Geometry check sheet. Reference: the model listing, model coordinates, mm. Give positions to 0.01 mm unless a question says otherwise; leave off trailing zeros. Order: outer loops, then holes, each group sorted by start corner. A loop starts at its lowest first (then second) coordinate and runs counter-clockwise, first axis right, second up. Notation, with made-up numbers: M 81.25,-25.75 L 94.25,-25.75 A28 cw 94.25,-2.75 Z; hole C 39,35 d10. An arc over 180 degrees is marked long. Answer as CSV lines item,"result". Start each with the question number.
```python
from build123d import *

# Parameters (mm, degrees)
F0_W     = 50
F0_H     = 70
F0_R     = 3
F1_DEPTH = 8
F2_SIZE  = 2
F3_SIZE  = 5


with BuildPart() as f1:
    # F0 (on Front) → F1 (new body)
    with BuildSketch(Plane.XZ):
        with Locations((-5.015146, 9.995409)):
            Rectangle(F0_W, F0_H)
        with Locations((-10.015146, 4.995409)):
            Circle(F0_R, mode=Mode.SUBTRACT)
        with Locations((11.984854, -17.004591)):
            Circle(F0_R, mode=Mode.SUBTRACT)
        with Locations((8.984854, 4.995409)):
            Circle(F0_R, mode=Mode.SUBTRACT)
        with Locations((11.984854, 36.995409)):
            Circle(F0_R, mode=Mode.SUBTRACT)
    extrude(amount=F1_DEPTH)

    # F2
    f2_edges = [f1.edges().sort_by_distance(p)[0] for p in [
        (-13.015146, -8, 4.995409),
        (5.984854, -8, 4.995409),
    ]]
    chamfer(f2_edges, length=F2_SIZE)

    # F3
    f3_edges = [f1.edges().sort_by_distance(p)[0] for p in [
        (19.984854, -4, 44.995409),
        (19.984854, -4, -25.004591),
        (-30.015146, -4, 44.995409),
        (-30.015146, -4, -25.004591),
    ]]
    chamfer(f3_edges, length=F3_SIZE)


solid = f1.part
```
Item 1: Section check B-B on y = -4.75. Record the boundary of the cut face in (x, z), then the cut area to 3 significant figures.
Item 2: Draft check along X on faces 1 (the face through (-13.14, -6.13, 5.13)), 2 (the face through (-30.015, -4, 10)), 3 (the face through (19.985, -4, 10)). Enter one of: pulls with the +X half, pulls with the -X half, needs draft (parallel to the pull), parting line crosses it, or undercut.
Item 3: Section check A-A on z = -18.5. Record the boundary of the cut face in (x, y), then the cut area to 3 significant figures.
Item 4: Scan lines: line 1 along X through (y, z) = (-7.5, 7); line 2 along X through (y, z) = (-5.5, 6); line 3 along Z through (x, y) = (11, -1.5). Record each from-to range of solid material in increasing order.
Item 5: Section check C-C on x = 10.5. Give the number of separate pieces and of enclosed holes in the cut face, then the cut area to 3 significant figures.
Numbers:
1,outline,"M -30.02,-20 L -25.02,-25 L 14.98,-25 L 19.98,-20 L 19.98,40 L 14.98,45 L -25.02,45 L -30.02,40 Z; hole C -10.02,5 d6; hole C 8.98,5 d6; hole C 11.98,-17 d6; hole C 11.98,37 d6"
1,area,"3,340 mm2"
2,face 1,"undercut"
2,face 2,"pulls with the -X half"
2,face 3,"pulls with the +X half"
3,outline,"M -30.02,-8 L 9.38,-8 L 9.38,0 L -30.02,0 Z; M 14.59,-8 L 19.98,-8 L 19.98,0 L 14.59,0 Z"
3,area,"358 mm2"
4,line 1,"-30.02 to -14.04, -5.99 to 4.96, 13.01 to 19.98"
4,line 2,"-30.02 to -12.84, -7.19 to 6.16, 11.81 to 19.98"
4,line 3,"-25 to -19.84, -14.17 to 2.77, 7.22 to 34.16, 39.83 to 45"
5,separate pieces,"4"
5,enclosed holes,"0"
5,area,"431 mm2"
